Design review of the part built by this model. Coordinates are the model's own, in mm. Face numbers are marked on the shaded views. A direction names the side the tool comes from. Coordinates: 2 decimals unless noted, no trailing zeros. Write each loop counter-clockwise with the first axis right and the second up, starting at its lowest first coordinate (ties: lowest second). Pieces come first, ordered by that corner, then holes.
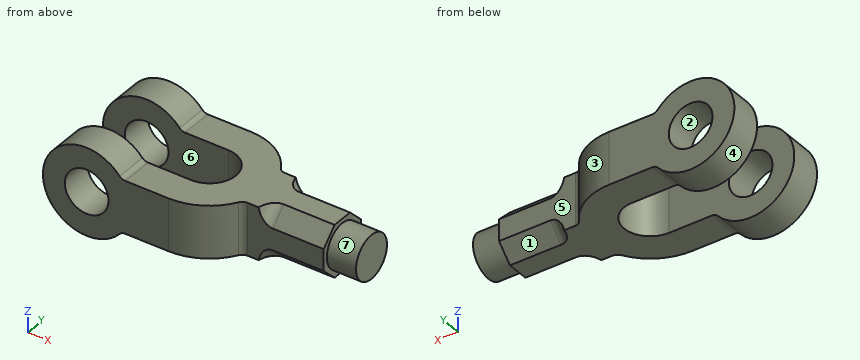
```python
from build123d import *

# Parameters (mm, degrees)
CROQUIS2_R              = 15
SALIENTE_EXTRUIR1_DEPTH = 40
CROQUIS3_W              = 99.474281043
CROQUIS3_H              = 36
CORTAR_EXTRUIR1_DEPTH   = 40
SALIENTE_EXTRUIR2_DEPTH = 36
SALIENTE_EXTRUIR3_DEPTH = 45
CROQUIS8_R              = 15
SALIENTE_EXTRUIR4_DEPTH = 20
REDONDEO1_R             = 10
REDONDEO2_R             = 5
REDONDEO3_R             = 5


with BuildPart() as part:
    # Croquis2 → Saliente-Extruir1 (new, symmetric)
    with BuildSketch(Plane(origin=(0, 0, 0), x_dir=(1, 0, 0), z_dir=(0, 1, 0))):
        with BuildLine():
            Line((24, -18), (56, -18))
            Line((56, -18), (56, 18))
            Line((56, 18), (24, 18))
            ThreePointArc((24, 18), (-30, 0), (24, -18))
        make_face()
        with Locations(Location((0, 0, 0), (0, 0, 270))):
            Circle(CROQUIS2_R, mode=Mode.SUBTRACT)
    extrude(amount=SALIENTE_EXTRUIR1_DEPTH, both=True)

    # Croquis3 → Cortar-Extruir1 (cut, symmetric)
    with BuildSketch(Plane.XY):
        with Locations((15.580182786, 0)):
            Rectangle(CROQUIS3_W, CROQUIS3_H)
    extrude(amount=CORTAR_EXTRUIR1_DEPTH, both=True, mode=Mode.SUBTRACT)


with BuildPart() as cortar_extruir1_piece_1:
    # of the separate pieces the step leaves, piece 1, a body of its own (cortar_extruir1_pieces)
    add(part.part.solids().sort_by_distance((24, -18, 18))[0])



with BuildPart() as cortar_extruir1_piece_2:
    # of the separate pieces the step leaves, piece 2, a body of its own (cortar_extruir1_pieces)
    add(part.part.solids().sort_by_distance((24, 40, 18))[0])


with BuildPart() as cortar_extruir1_piece_1_1:
    add(cortar_extruir1_piece_1.part)

    add(cortar_extruir1_piece_2.part)  # Saliente-Extruir2 merges Cortar-Extruir1 piece 2
    # Croquis5 → Saliente-Extruir2 (add)
    with BuildSketch(Plane.XY.offset(18)):
        with BuildLine():
            Line((91.721142199, 18), (102, 18))
            Line((102, 18), (102, -18))
            Line((102, -18), (91.721142199, -18))
            ThreePointArc((91.721142199, -18), (76.976176963, -34.058772732), (56, -40))
            Line((56, -40), (56, -18))
            ThreePointArc((56, -18), (74, 0), (56, 18))
            Line((56, 18), (56, 40))
            ThreePointArc((56, 40), (76.976176963, 34.058772732), (91.721142199, 18))
        make_face()
    extrude(amount=-SALIENTE_EXTRUIR2_DEPTH)

    # Croquis7 → Saliente-Extruir3 (add)
    with BuildSketch(Plane(origin=(102, 0, 0), x_dir=(0, 0, -1), z_dir=(1, 0, 0))):
        Polygon((-7.455844123, 18), (-18, 7.455844123), (-18, -7.455844123), (-7.455844123, -18), (7.455844123, -18), (18, -7.455844123), (18, 7.455844123), (7.455844123, 18), align=None)
    extrude(amount=SALIENTE_EXTRUIR3_DEPTH)

    # Croquis8 → Saliente-Extruir4 (add)
    with BuildSketch(Plane(origin=(147, 0, 0), x_dir=(0, 0, -1), z_dir=(1, 0, 0))):
        Circle(CROQUIS8_R)
    extrude(amount=SALIENTE_EXTRUIR4_DEPTH)

    # Redondeo1
    # the kernel refuses this fillet: 10 mm, written as the material it adds along each edge
    with BuildSketch(Plane(origin=(102, 35.67766953, -10.221825407), x_dir=(1, 0, 0), z_dir=(0, -0.7071067811865477, 0.7071067811865475))) as redondeo1_piece_1_section:
        with BuildLine():
            CenterArc((REDONDEO1_R, REDONDEO1_R), REDONDEO1_R, 180, 90)
            Line((0, REDONDEO1_R), (0, 0))
            Line((0, 0), (REDONDEO1_R, 0))
        make_face()
    redondeo1_piece_1 = extrude(amount=64.911688245, mode=Mode.PRIVATE)
    redondeo1_piece_1 = split(redondeo1_piece_1, bisect_by=Plane(origin=(104.775136412, 13.729156697, 18), z_dir=(0, 0, -1)), keep=Keep.TOP, mode=Mode.PRIVATE)
    redondeo1_piece_1 = split(redondeo1_piece_1, bisect_by=Plane(origin=(104.775136412, 18, 13.729156697), z_dir=(0, -1, 0)), keep=Keep.TOP, mode=Mode.PRIVATE)
    add(redondeo1_piece_1)
    with BuildSketch(Plane(origin=(102, -10.221825407, -35.67766953), x_dir=(1, 0, 0), z_dir=(0, 0.7071067811865475, 0.7071067811865476))) as redondeo1_piece_2_section:
        with BuildLine():
            CenterArc((REDONDEO1_R, REDONDEO1_R), REDONDEO1_R, 180, 90)
            Line((0, REDONDEO1_R), (0, 0))
            Line((0, 0), (REDONDEO1_R, 0))
        make_face()
    redondeo1_piece_2 = extrude(amount=64.911688245, mode=Mode.PRIVATE)
    redondeo1_piece_2 = split(redondeo1_piece_2, bisect_by=Plane(origin=(104.775136412, 18, -13.729156697), z_dir=(0, -1, 0)), keep=Keep.TOP, mode=Mode.PRIVATE)
    redondeo1_piece_2 = split(redondeo1_piece_2, bisect_by=Plane(origin=(104.775136412, 13.729156697, -18), z_dir=(0, 0, 1)), keep=Keep.TOP, mode=Mode.PRIVATE)
    add(redondeo1_piece_2)
    with BuildSketch(Plane(origin=(102, -35.67766953, 10.221825407), x_dir=(1, 0, 0), z_dir=(0, 0.7071067811865477, -0.7071067811865475))) as redondeo1_piece_3_section:
        with BuildLine():
            CenterArc((REDONDEO1_R, REDONDEO1_R), REDONDEO1_R, 180, 90)
            Line((0, REDONDEO1_R), (0, 0))
            Line((0, 0), (REDONDEO1_R, 0))
        make_face()
    redondeo1_piece_3 = extrude(amount=64.911688245, mode=Mode.PRIVATE)
    redondeo1_piece_3 = split(redondeo1_piece_3, bisect_by=Plane(origin=(104.775136412, -18, -13.729156697), z_dir=(0, 1, 0)), keep=Keep.TOP, mode=Mode.PRIVATE)
    redondeo1_piece_3 = split(redondeo1_piece_3, bisect_by=Plane(origin=(104.775136412, -13.729156697, -18), z_dir=(0, 0, 1)), keep=Keep.TOP, mode=Mode.PRIVATE)
    add(redondeo1_piece_3)
    with BuildSketch(Plane(origin=(102, 10.221825407, 35.67766953), x_dir=(0, -0.7071067811865476, 0.7071067811865476), z_dir=(0, -0.7071067811865476, -0.7071067811865476))) as redondeo1_piece_4_section:
        with BuildLine():
            CenterArc((REDONDEO1_R, -REDONDEO1_R), REDONDEO1_R, 90, 90)
            Line((0, -REDONDEO1_R), (0, 0))
            Line((0, 0), (REDONDEO1_R, 0))
        make_face()
    redondeo1_piece_4 = extrude(amount=64.911688245, mode=Mode.PRIVATE)
    redondeo1_piece_4 = split(redondeo1_piece_4, bisect_by=Plane(origin=(104.775136413, -13.729156697, 18), z_dir=(0, 0, -1)), keep=Keep.TOP, mode=Mode.PRIVATE)
    redondeo1_piece_4 = split(redondeo1_piece_4, bisect_by=Plane(origin=(104.775136413, -18, 13.729156697), z_dir=(0, 1, 0)), keep=Keep.TOP, mode=Mode.PRIVATE)
    add(redondeo1_piece_4)

    # Redondeo2
    redondeo2_edges = [cortar_extruir1_piece_1_1.edges().sort_by_distance(p)[0] for p in [
        (91.721142199, 18, 0),
        (91.721142199, -18, 0),
    ]]
    fillet(redondeo2_edges, radius=REDONDEO2_R)

    # Redondeo3
    redondeo3_edges = [cortar_extruir1_piece_1_1.edges().sort_by_distance(p)[0] for p in [
        (24, -29, 18),
        (24, -29, -18),
        (24, 29, -18),
        (24, 29, 18),
    ]]
    fillet(redondeo3_edges, radius=REDONDEO3_R)


solid = cortar_extruir1_piece_1_1.part
```
(1) Consider section C-C (y = 0). Give the boundary of the cut face in (x, z).
(2) For the marked faces 5, 6 and 7, list the 3-axis set-ups (+Z, -Z, +X, -X, +Y, -Y) from which the entire face can be reached by the end or side of a thin tool; tool diameter is ignored.
(3) Consider section A-A (z = 0). Give the boundary of the cut face in (x, y), plus the area to 3 significant figures.
(4) Consider section B-B (x = 49.5). Give the boundary of the cut face in (y, z).
(5) Insertion check: pin 1 Ø6 at (x, z) = (91.5, 22) entering from +Y; pin 2 Ø1.5 at (y, z) = (2.5, -10) entering from -X; pin 3 Ø12 at (y, z) = (0, -2) entering from -X; pin 4 Ø24 at (x, y) = (57, 20) entering from +Z. Each pin has a flat end and moves straight along its axis. Give the tip position at first contact, or say it passes through.
(6) Mouldability with a two-part tool opening along X and no side actions: class the marked faces 1, 2, 3 and 4 as +X half, -X half, draft (parallel to the pull), parting line (faces both ways), or undercut.
(7) Consider section D-D (x = 0). Give the boundary of the cut face in (y, z).
(8) Wall thickness on line 1 (Y direction, x = 54.5, z = 14.5); line 2 (Z direction, x = 0, y = -28); line 3 (Y direction, x = 60, z = -7.5): over which ranges is each line inside the solid? List them lowest first.
Results:
1. outline: (74, -18) - (147, -18) - (147, -15) - (167, -15) - (167, 15) - (147, 15) - (147, 18) - (74, 18) - close
2. face 5: +Z, -Z, +X, +Y
2. face 6: +Z, -Z, -X
2. face 7: +X
3. outline: (-30, -40) - (-15, -40) - (-15, -18) - (-30, -18) - close; (-30, 18) - (-15, 18) - (-15, 40) - (-30, 40) - close; (15, -40) - (56, -40) arc R40 ccw to (90.38, -20.44) arc R5 cw to (94.68, -18) - (147, -18) - (147, -15) - (167, -15) - (167, 15) - (147, 15) - (147, 18) - (94.68, 18) arc R5 cw to (90.38, 20.44) arc R40 ccw to (56, 40) - (15, 40) - (15, 18) - (56, 18) arc R18 cw to (56, -18) - (15, -18) - close
3. area: 6,960 mm2
4. outline: (-40, -18) - (-18, -18) - (-18, 18) - (-40, 18) - close; (18, -18) - (40, -18) - (40, 18) - (18, 18) - close
5. pin 1: passes through
5. pin 2: stops at x = 73.7
5. pin 3: stops at x = 72.97
5. pin 4: stops at z = 18
6. face 1: draft
6. face 2: undercut
6. face 3: +X half
6. face 4: parting line
7. outline: (-40, -30) - (-18, -30) - (-18, -15) - (-40, -15) - close; (-40, 15) - (-18, 15) - (-18, 30) - (-40, 30) - close; (18, -30) - (40, -30) - (40, -15) - (18, -15) - close; (18, 15) - (40, 15) - (40, 30) - (18, 30) - close
8. line 1: y = -40 to -18, 18 to 40
8. line 2: z = -30 to -15, 15 to 30
8. line 3: y = -39.8 to -17.55, 17.55 to 39.8
